from build123d import *

# Parameters (mm, degrees)
F0_R      = 14.5993643937
F1_DEPTH  = 50.8
F2_R      = 14.478
F3_T      = -2.54
F4_W      = 31.7054085236
F4_H      = 7.25655691
F4_R      = 0.1213643937
F1_FACE_R = 0.1213643937
F3_FACE_R = 0.1213643937
F5_DEPTH  = 17.526
F6_R      = 3.048
F7_DEPTH  = 23.876
F8_R      = 3.048
F9_DEPTH  = 37.592


with BuildPart() as f1:
    # F0 (on Top) → F1 (new body)
    with BuildSketch(Plane.XY):
        Circle(F0_R)
    extrude(amount=F1_DEPTH)

    # F2
    f2_edges = [f1.edges().sort_by_distance(p)[0] for p in [
        (-14.599364, 0, 50.8),
    ]]
    fillet(f2_edges, radius=F2_R)

    # F3
    f3_openings = [f1.faces().sort_by_distance(p)[0] for p in [
        (0, 0, 0),
    ]]
    offset(amount=F3_T, openings=f3_openings)

    # F4 (on face) + F1_face (on face) + F3_face (on face) → F5 (cut)
    with BuildSketch(Plane.XY.offset(50.8)):
        Rectangle(F4_W, F4_H)
        Circle(F4_R, mode=Mode.SUBTRACT)
    with BuildSketch(Plane.XY.offset(50.8)):
        Circle(F1_FACE_R)
    with BuildSketch(Plane(origin=(0, 0, 48.26), x_dir=(1, 0, 0), z_dir=(0, 0, -1))):
        Circle(F3_FACE_R)
    extrude(amount=-F5_DEPTH, dir=(0, 0, 1), mode=Mode.SUBTRACT)

    # F6 (on Front) → F7 (cut)
    with BuildSketch(Plane.XZ):
        with Locations((0, 28.448)):
            Circle(F6_R)
    extrude(amount=-F7_DEPTH, mode=Mode.SUBTRACT)

    # F8 (on Front) → F9 (cut)
    with BuildSketch(Plane.XZ):
        with Locations((0, 28.448)):
            Circle(F8_R)
    extrude(amount=F9_DEPTH, mode=Mode.SUBTRACT)


solid = f1.part
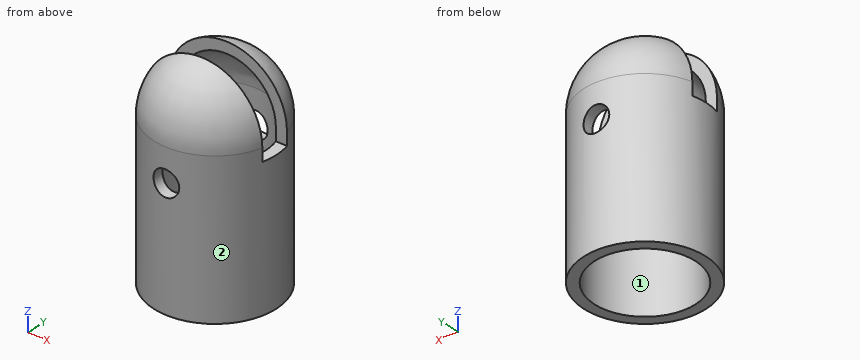
Work out the finished part from the listing and answer in its coordinate system (mm). Face numbers are marked on the shaded views. Give positions to 0.01 mm unless a question says otherwise; leave off trailing zeros. Order: outer loops, then holes, each group sorted by start corner. A loop starts at its lowest first (then second) coordinate and runs counter-clockwise, first axis right, second up. Notation, with made-up numbers: M -23,0.5 L 4,0.5 A14 cw 4,24.5 Z; hole C 64.25,-18.75 d3. An arc over 180 degrees is marked long. Return JSON: item names as keys, results as strings.
Q1. Find section C-C, the plane x = 0. State how many separate pieces and enclosed holes the cut face has, and give its area (3 significant figures).
Answer below:
{"separate pieces": "4", "enclosed holes": "0", "area": "241 mm^2"}
Q2. Each of these flat-tipped pins is pushed along its axis until it touches: pin 1 (1.5 mm diameter, centred on x = 13.5, y = -1.5, fed in from +Z); pin 2 (2 mm diameter, centred on x = 5.5, z = 37, fed in from -Y); pin 3 (5 mm diameter, centred on x = 0, z = 28.448, fed in from +Y); pin 4 (5 mm diameter, centred on x = 0, z = 42, fed in from -Y). Where does it stop, or does it pass through?
Answer below:
{"pin 1": "stops at z = 33.27", "pin 2": "stops at y = -13.87", "pin 3": "passes through", "pin 4": "stops at y = -14.25"}
Q3. Find section A-A, the plane z = 34. Write down the section's boundary in (x, y), and give its area (3 significant figures).
Answer below:
{"outline": "M -14.14,-3.63 A14.6 ccw 14.14,-3.63 L 11.5,-3.63 A12.06 cw -11.5,-3.63 Z; M -14.14,3.63 L -11.5,3.63 A12.06 cw 11.5,3.63 L 14.14,3.63 A14.6 ccw Z", "area": "175 mm^2"}
Q4. Find the intervals of material crossed by line 1 along Y through (x, z) = (0, 18.5); line 2 along X through (y, z) = (2, 23); line 3 along X through (y, z) = (-10.5, 12), in increasing order. Write a range as [from, to].
Answer below:
{"line 1": "y = [-14.6, -12.06], [12.06, 14.6]", "line 2": "x = [-14.46, -11.89], [11.89, 14.46]", "line 3": "x = [-10.14, -5.93], [5.93, 10.14]"}
Q5. Find section B-B, the plane y = 0. Write down the section's boundary in (x, z), and give its area (3 significant figures).
Answer below:
{"outline": "M -14.6,0 L -12.06,0 L -12.06,33.27 L -14.6,33.27 Z; M 12.06,0 L 14.6,0 L 14.6,33.27 L 12.06,33.27 Z", "area": "169 mm^2"}
Q6. The mould has two halves that part along X. Classify the marked faces 1 and 2: pulls with the +X half, pulls with the -X half, needs draft (parallel to the pull), parting line crosses it, or undercut.
Answer below:
{"face 1": "undercut", "face 2": "parting line crosses it"}
